Read the model definition and answer for the solid it produces. Units are mm, in the model's axes. Face numbers are marked on the shaded views. Give positions to 0.01 mm unless a question says otherwise; leave off trailing zeros. Order: outer loops, then holes, each group sorted by start corner. A loop starts at its lowest first (then second) coordinate and runs counter-clockwise, first axis right, second up.
```python
from build123d import *

# Parameters (mm, degrees)
SKETCH1_R           = 4.25
BOSS_EXTRUDE1_DEPTH = 4.2
CHAMFER1_SIZE       = 0.75


with BuildPart() as part:
    # Sketch1 → Boss-Extrude1 (new, symmetric)
    with BuildSketch(Plane.XY):
        Polygon((0, 9.237604307), (-8, 4.618802154), (-8, -4.618802154), (0, -9.237604307), (8, -4.618802154), (8, 4.618802154), align=None)
        Circle(SKETCH1_R, mode=Mode.SUBTRACT)
    extrude(amount=BOSS_EXTRUDE1_DEPTH, both=True)

    # Sketch4 → Cut-Revolve5 (revolve, cut)
    with BuildSketch(Plane(origin=(0, 0, 0), x_dir=(0, 0, -1), z_dir=(1, 0, 0))):
        Polygon((3.48546882, 9.237604307), (4.2, 8), (4.2, 9.237604307), align=None)
    revolve(axis=Axis((0, 0, 0), (0, 0, -1)), mode=Mode.SUBTRACT)

    # Sketch5 → Cut-Revolve6 (revolve, cut)
    with BuildSketch(Plane(origin=(0, 0, 0), x_dir=(0, 0, -1), z_dir=(1, 0, 0))):
        Polygon((-3.48546882, 9.237604307), (-4.2, 8), (-4.2, 9.237604307), align=None)
    revolve(axis=Axis((0, 0, 0), (0, 0, 1)), mode=Mode.SUBTRACT)

    # Chamfer1
    chamfer1_edges = [part.edges().sort_by_distance(p)[0] for p in [
        (-4.25, 0, -4.2),
        (-4.25, 0, 4.2),
    ]]
    chamfer(chamfer1_edges, length=CHAMFER1_SIZE)


solid = part.part
```
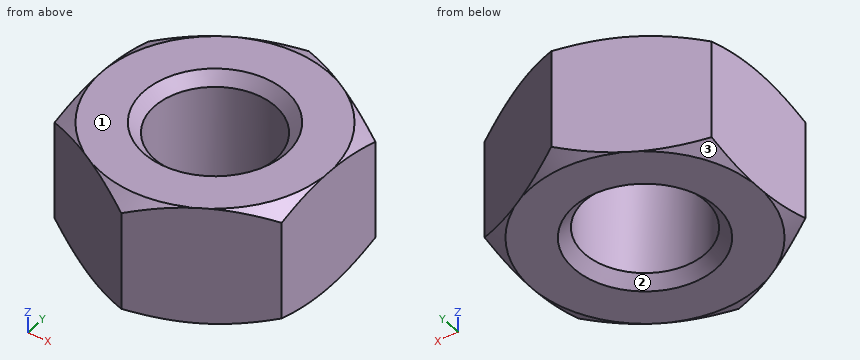
1) The part is cut by section A-A on z = 1. Determine the outline of the cut face in (x, y), and give its area (3 significant figures).
Final values:
outline: (-8, -4.62) - (0, -9.24) - (8, -4.62) - (8, 4.62) - (0, 9.24) - (-8, 4.62) - close; hole circle Ø8.5 at (0, 0)
area: 165 mm2
2) For a pull along X with two mould halves and no side action, classify the marked faces 1, 2 and 3 as released by +X, released by -X, zero draft, split by the parting line, or undercut.
Final values:
face 1: zero draft
face 2: undercut
face 3: released by -X
3) Consider L1, parallel to X at y = 2, z = 3; L2, parallel to X at y = -3, z = -1.5; L3, parallel to Y at x = 1, z = -4. Determine where each line is inside the solid, lowest interval first.
Final values:
L1: x = -8 to -3.75, 3.75 to 8
L2: x = -8 to -3.01, 3.01 to 8
L3: y = -8.29 to -4.69, 4.69 to 8.29
4) Given pin 1 (5 mm diameter, centred on x = 5, z = -1, fed in from -Y); pin 2 (4 mm diameter, centred on x = -5, z = 2, fed in from -Y); pin 3 (2 mm diameter, centred on x = -3.5, z = 3, fed in from +Y), each flat-ended and moving along its own axis, determine where each tip first touches the part or whether it passes through.
Final values:
pin 1: stops at y = -7.79
pin 2: stops at y = -7.51
pin 3: stops at y = 7.79
